from build123d import *

# Parameters (mm, degrees)
ESQUISSE1_W             = 27
ESQUISSE1_H             = 6
ESQUISSE1_R             = 1.65
BOSS_EXTRU_1_DEPTH      = 3.15
ESQUISSE3_W             = 12
ESQUISSE3_H             = 6
BOSS_EXTRU_2_DEPTH      = 5.5
ESQUISSE4_W             = 10
ESQUISSE4_H             = 2.5
ENL_V_MAT_EXTRU_1_DEPTH = 10
ESQUISSE5_R             = 0.49
ENL_V_MAT_EXTRU_2_DEPTH = 1.5
CHANFREIN1_SIZE         = 1.3


with BuildPart() as part:
    # Esquisse1 → Boss.-Extru.1 (new body)
    with BuildSketch(Plane.XY):
        with Locations((-13.5, 3)):
            Rectangle(ESQUISSE1_W, ESQUISSE1_H)
        with Locations((-24, 3)):
            Circle(ESQUISSE1_R, mode=Mode.SUBTRACT)
        with Locations((-3, 3)):
            Circle(ESQUISSE1_R, mode=Mode.SUBTRACT)
    extrude(amount=BOSS_EXTRU_1_DEPTH)

    # Esquisse3 → Boss.-Extru.2 (add)
    with BuildSketch(Plane.XY.offset(3.15)):
        with Locations((-13.5, 3)):
            Rectangle(ESQUISSE3_W, ESQUISSE3_H)
    extrude(amount=BOSS_EXTRU_2_DEPTH)

    # Esquisse4 → Enlèv. mat.-Extru.1 (cut)
    with BuildSketch(Plane.XY.offset(8.65)):
        with Locations((-13.5, 3)):
            Rectangle(ESQUISSE4_W, ESQUISSE4_H)
    extrude(amount=-ENL_V_MAT_EXTRU_1_DEPTH, mode=Mode.SUBTRACT)

    # Esquisse5 → Enlèv. mat.-Extru.2 (cut)
    with BuildSketch(Plane.XY.offset(8.65)):
        with Locations((-9.54, 4.785)):
            Circle(ESQUISSE5_R)
        with Locations((-17.46, 1.215)):
            Circle(ESQUISSE5_R)
    extrude(amount=-ENL_V_MAT_EXTRU_2_DEPTH, mode=Mode.SUBTRACT)

    # Chanfrein1
    chanfrein1_edges = [part.edges().sort_by_distance(p)[0] for p in [
        (-4.65, 3, 0),
        (-25.65, 3, 0),
    ]]
    chamfer(chanfrein1_edges, length=CHANFREIN1_SIZE)


solid = part.part
Read the model definition and answer for the solid it produces. Units are mm, in the model's axes. A direction names the side the tool comes from. Round coordinates to 2 decimals unless told otherwise and drop trailing zeros. Write each loop counter-clockwise with the first axis right and the second up, starting at its lowest first coordinate (ties: lowest second). Pieces come first, ordered by that corner, then holes. Notation, with made-up numbers: M -4,-16.75 L 37,-16.75 A22 cw 37,12.25 Z; hole C 72.5,2 d3. An arc over 180 degrees is marked long. Use a Markdown table: item, result.
1) A tool of negligible diameter and unlimited length cuts with its end or side. For faces 1 (the flat face through (-17.5, 1.2, 7.15)), 2 (the flat face through (-18.5, 3, 4)), 3 (the flat face through (-5, 4, 3.15)), 4 (the flat face through (-14, 0, 3)), 5 (the flat face through (-22, 4, 3.15)), from which of +Z, -Z, +X, -X, +Y, -Y can it reach the whole face along a straight path? Write none if from no direction.
Answers follow:
| item | result |
|---|---|
| face 1 | +Z |
| face 2 | +Z, -Z |
| face 3 | +Z, +X, +Y, -Y |
| face 4 | +Z, -Z, +X, -X, -Y |
| face 5 | +Z, -X, +Y, -Y |
2) The part is cut by section B-B (y = 3). Write down the section's boundary in (x, z), plus the area to 3 significant figures.
Answers follow:
| item | result |
|---|---|
| outline | M -27,0 L -26.95,0 L -25.65,1.3 L -25.65,3.15 L -27,3.15 Z; M -22.35,1.3 L -21.05,0 L -18.5,0 L -18.5,8.65 L -19.5,8.65 L -19.5,3.15 L -22.35,3.15 Z; M -8.5,0 L -5.95,0 L -4.65,1.3 L -4.65,3.15 L -7.5,3.15 L -7.5,8.65 L -8.5,8.65 Z; M -1.35,1.3 L -0.05,0 L 0,0 L 0,3.15 L -1.35,3.15 Z |
| area | 40.4 mm2 |
3) Flat-ended cylindrical pins translate along their axes: pin 1 (3 mm diameter, centred on y = 2, z = 5.5, fed in from +X); pin 2 (3 mm diameter, centred on x = -25, y = 2.5, fed in from +Z); pin 3 (1.8 mm diameter, centred on x = -3.5, y = 3, fed in from +Z). Find the tip coordinate at first contact, or state that the pin passes through.
Answers follow:
| item | result |
|---|---|
| pin 1 | stops at x = -7.5 |
| pin 2 | stops at z = 3.15 |
| pin 3 | passes through |
4) Straight lines are drawn through the part: line 1 along X through (y, z) = (2.05, 3.25); line 2 along Y through (x, z) = (-12.75, 7.75); line 3 along Y through (x, z) = (-3, 2.65). For each, find the intervals that lie inside material, in ascending order. Write a range as [from, to].
Answers follow:
| item | result |
|---|---|
| line 1 | x = [-19.5, -18.5], [-8.5, -7.5] |
| line 2 | y = [0, 1.75], [4.25, 6] |
| line 3 | y = [0, 1.35], [4.65, 6] |
5) The part is cut by section D-D (z = 0.5). Write down the section's boundary in (x, y).
Answers follow:
| item | result |
|---|---|
| outline | M -27,0 L 0,0 L 0,6 L -27,6 Z; hole C -24,3 d4.9; hole M -18.5,1.75 L -8.5,1.75 L -8.5,4.25 L -18.5,4.25 Z; hole C -3,3 d4.9 |
6) For a pull along X with two mould halves and no side action, classify faces 6 (the flat face through (0, 3, 2)), 7 (the flat face through (-13.6, 4.4, 8.65)), 8 (the cylindrical face through (-25.65, 3.07, 2.21)) as pulls with the +X half, pulls with the -X half, needs draft (parallel to the pull), parting line crosses it, or undercut.
Answers follow:
| item | result |
|---|---|
| face 6 | pulls with the +X half |
| face 7 | needs draft |
| face 8 | undercut |
7) The part is cut by section C-C (z = 4). Write down the section's boundary in (x, y), plus the area to 3 significant figures.
Answers follow:
| item | result |
|---|---|
| outline | M -19.5,0 L -7.5,0 L -7.5,6 L -19.5,6 Z; hole M -18.5,1.75 L -8.5,1.75 L -8.5,4.25 L -18.5,4.25 Z |
| area | 47.0 mm2 |
8) The part is cut by section A-A (x = -17.46). Write down the section's boundary in (y, z) (3 decimals), plus the area to 3 significant figures.
Answers follow:
| item | result |
|---|---|
| outline | M 0,0 L 1.75,0 L 1.75,8.65 L 1.705,8.65 L 1.705,7.15 L 0.725,7.15 L 0.725,8.65 L 0,8.65 Z; M 4.25,0 L 6,0 L 6,8.65 L 4.25,8.65 Z |
| area | 28.8 mm2 |
